Part print with two shaded views. Sizes in mm from the minimum x, y, z corner. A direction names the side the tool comes from. Give positions to 0.01 mm unless a question says otherwise; leave off trailing zeros. Loops run counter-clockwise (first coordinate to the right, second up) from the corner with the lowest first, then second, coordinate; pieces in that order, holes last. Notation, with made-up numbers: (47, 40.25) -> (68, 40.25) arc R18 cw to (68, 45.25) -> close; hole circle Ø7 at (-16.75, 54). An arc over 180 degrees is marked (long way). One line per question, with ' | ' between items. Start each with the question number.
(1) Drill centre lines: L1, parallel to Y at x = 50, z = 311; L2, parallel to Y at x = 169, z = 171; L3, parallel to Y at x = 50.8, z = 306.25. Where is each one in solid material? Low to high. Write a range as from..to.
(2) Slice it at D-D, the plane z = 84. Write the cut outline in (x, y).
(3) Slice it at B-B, the plane z = 310. Write the cut outline in (x, y), then the cut area to 3 significant figures.
(4) Slice it at C-C, the plane x = 263.5. Write the cut outline in (y, z).
(5) Slice it at A-A, the plane x = 50.8. Write the cut outline in (y, z).
(6) Flat gauge pins, fed straight in: pin 1 Ø7.5 at (y, z) = (60, 308.5) entering from +X; pin 2 Ø23 at (x, y) = (50.8, 108.966) entering from -Z; pin 3 Ø7.5 at (y, z) = (72, 307.5) entering from -X; pin 4 Ø23 at (x, y) = (54.5, 63.5) entering from -Z. Where does each tip first touch, or does it go through?
(7) 3-axis set-ups, long thin cutter, end or side, ignore diameter. For the marked faces 1 and 2: which of +Z, -Z, +X, -X, +Y, -Y reach the whole face in a straight line?
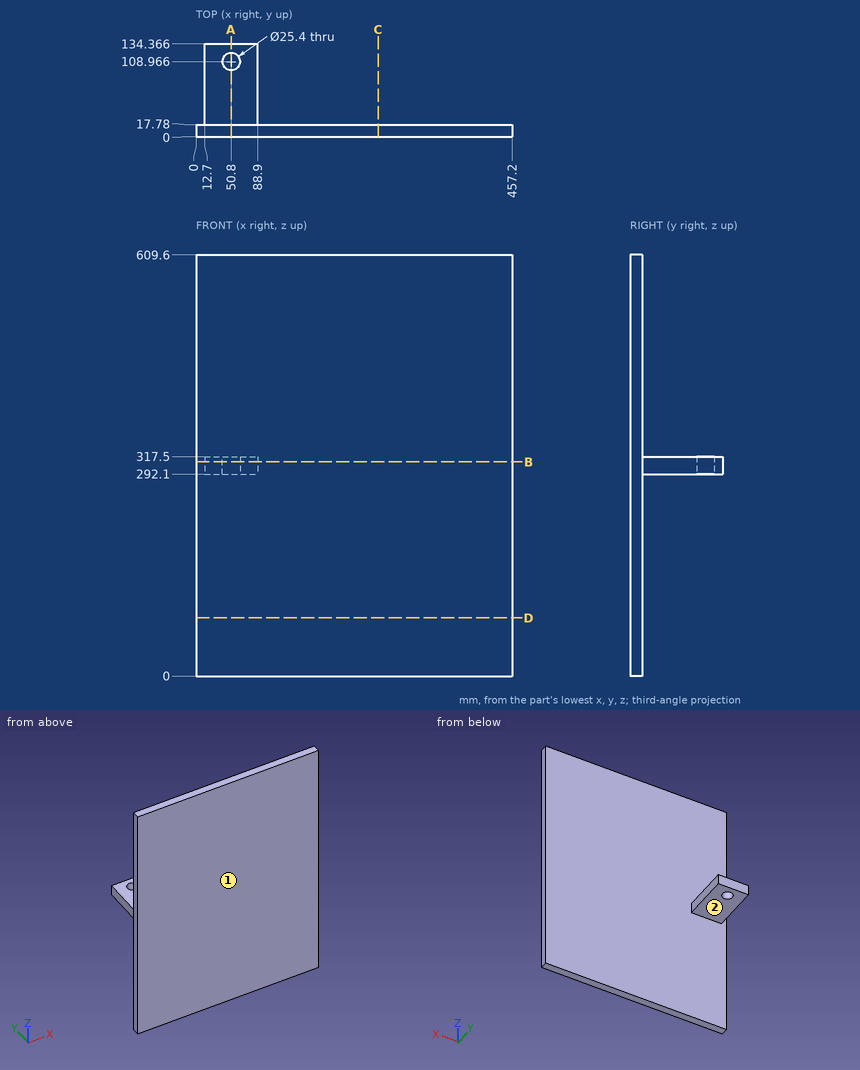
Final values:
1) L1: 0..96.29, 121.64..134.37 | L2: 0..17.78 | L3: 0..96.27, 121.67..134.37
2) outline: (0, 0) -> (457.2, 0) -> (457.2, 17.78) -> (0, 17.78) -> close
3) outline: (0, 0) -> (457.2, 0) -> (457.2, 17.78) -> (88.9, 17.78) -> (88.9, 134.37) -> (12.7, 134.37) -> (12.7, 17.78) -> (0, 17.78) -> close; hole circle Ø25.4 at (50.8, 108.97) | area: 16,500 mm2
4) outline: (0, 0) -> (17.78, 0) -> (17.78, 609.6) -> (0, 609.6) -> close
5) outline: (0, 0) -> (17.78, 0) -> (17.78, 292.1) -> (96.27, 292.1) -> (96.27, 317.5) -> (17.78, 317.5) -> (17.78, 609.6) -> (0, 609.6) -> close; (121.67, 292.1) -> (134.37, 292.1) -> (134.37, 317.5) -> (121.67, 317.5) -> close
6) pin 1: x = 88.9 | pin 2: through | pin 3: x = 12.7 | pin 4: z = 292.1
7) face 1: +Z, -Z, +X, -X, -Y | face 2: -Z, +X, -X, +Y
